```python
from build123d import *

# Parameters (mm, degrees)
BOSS_EXTRUDE1_DEPTH = 100
CUT_EXTRUDE1_DEPTH  = 50


with BuildPart() as part:
    # Sketch1 → Boss-Extrude1 (new body)
    with BuildSketch(Plane(origin=(0, 0, 0), x_dir=(1, 0, 0), z_dir=(0, 1, 0))):
        Polygon((-105.576923077, -23.605769231), (44.423076923, -23.605769231), (44.423076923, 56.394230769), (-18.173076923, 56.394230769), (-18.173076923, 36.394230769), (-40.576923077, 36.394230769), (-40.576923077, 16.394230769), (-60.576923077, 16.394230769), (-60.576923077, 37.644230769), (-80.576923077, 37.644230769), (-80.576923077, 56.394230769), (-105.576923077, 56.394230769), align=None)
    extrude(amount=-BOSS_EXTRUDE1_DEPTH)

    # Sketch3 → Cut-Extrude1 (cut)
    with BuildSketch(Plane(origin=(44.423076923, 0, 0), x_dir=(0, 0, -1), z_dir=(1, 0, 0))):
        Polygon((56.394230769, -25), (11.394230769, -52.073671681), (56.394230769, -75), align=None)
    extrude(amount=-CUT_EXTRUDE1_DEPTH, mode=Mode.SUBTRACT)


solid = part.part
```
Build history of the part. All positions in model axes, mm. A direction names the side the tool comes from. Coordinates: 2 decimals unless noted, no trailing zeros. Write each loop counter-clockwise with the first axis right and the second up, starting at its lowest first coordinate (ties: lowest second). Pieces come first, ordered by that corner, then holes.
1. Drop flat-ended pins along their axis: pin 1 (6 mm diameter, centred on x = -71.5, y = -50, fed in from -Z); pin 2 (6 mm diameter, centred on x = -53, y = -50, fed in from -Z); pin 3 (5.5 mm diameter, centred on y = -36.5, z = -49.5, fed in from +X). Give the stop position or say it passes through.
Answer block:
pin 1: stops at z = -37.64
pin 2: stops at z = -16.39
pin 3: stops at x = -5.58
2. Band-saw the part on A-A, the plane y = -18.5. Give the cut face in (x, z), and give its area (3 significant figures).
Answer block:
outline: (-105.58, -56.39) - (-80.58, -56.39) - (-80.58, -37.64) - (-60.58, -37.64) - (-60.58, -16.39) - (-40.58, -16.39) - (-40.58, -36.39) - (-18.17, -36.39) - (-18.17, -56.39) - (44.42, -56.39) - (44.42, 23.61) - (-105.58, 23.61) - close
area: 10,400 mm2
3. Pull direction X, two halves, no side cores. Call faces 4 (the flat face through (-60.577, -49, -27)), 5 (the flat face through (-32, -49, 23.606)), 6 (the flat face through (-105.577, -49, -17)): released by +X, released by -X, zero draft, split by the parting line, or undercut.
Answer block:
face 4: undercut
face 5: zero draft
face 6: released by -X
4. Band-saw the part on B-B, the plane z = -31.5. Give the cut face in (x, y).
Answer block:
outline: (-105.58, -100) - (-60.58, -100) - (-60.58, 0) - (-105.58, 0) - close; (-40.58, -100) - (44.42, -100) - (44.42, -62.32) - (-5.58, -62.32) - (-5.58, -39.98) - (44.42, -39.98) - (44.42, 0) - (-40.58, 0) - close
5. 3-axis set-ups, long thin cutter, end or side, ignore diameter. For faces 1 (the flat face through (-32, 0, -17)), 2 (the flat face through (19.773, -38.347, -34.209)), 3 (the flat face through (-29, -49, -36.394)): which of +Z, -Z, +X, -X, +Y, -Y reach the whole face in a straight line?
Answer block:
face 1: +Z, -Z, +X, -X, +Y
face 2: -Z, +X
face 3: -Z, +Y, -Y
6. Band-saw the part on C-C, the plane x = 31. Give the cut face in (y, z), and give its area (4 significant figures).
Answer block:
outline: (-100, -56.39) - (-75, -56.39) - (-52.07, -11.39) - (-25, -56.39) - (0, -56.39) - (0, 23.61) - (-100, 23.61) - close
area: 6,875 mm2
7. Drill centre lines: probe 1 along X at (y, z) = (-8, -26.5); probe 2 along X at (y, z) = (-46, -52); probe 3 along Z at (x, y) = (-23, -55.5). Where is each one in solid material? Low to high.
Answer block:
probe 1: x = -105.58 to -60.58, -40.58 to 44.42
probe 2: x = -105.58 to -80.58, -18.17 to -5.58
probe 3: z = -36.39 to 23.61
8. Band-saw the part on D-D, the plane x = -76.5. Give the cut face in (y, z), and give its area (4 significant figures).
Answer block:
outline: (-100, -37.64) - (0, -37.64) - (0, 23.61) - (-100, 23.61) - close
area: 6,125 mm2
